Design review of the part built by this model. Coordinates are the model's own, in mm. Round coordinates to 2 decimals unless told otherwise and drop trailing zeros. Order: outer loops, then holes, each group sorted by start corner. A loop starts at its lowest first (then second) coordinate and runs counter-clockwise, first axis right, second up. Notation, with made-up numbers: (-7.5, -10.75) - (29.5, -10.75) arc R21 ccw to (29.5, 2.25) - close; hole circle Ø3 at (53.5, -29). An arc over 180 degrees is marked (long way). Write item = value, one per line.
from build123d import *

# Parameters (mm, degrees)
F0_W    = 4
F0_H    = 2.5
F2_SIZE = 0.4


with BuildPart() as f1:
    # F0 (on Front) → F1 (revolve)
    with BuildSketch(Plane.XZ):
        with Locations((2, 3.75)):
            Rectangle(F0_W, F0_H)
    revolve(axis=Axis((1.361359, 0, 0), (1, 0, 0)))

    # F2
    f2_edges = [f1.edges().sort_by_distance(p)[0] for p in [
        (0, 0, -2.5),
        (4, 0, -2.5),
        (2, 0, 2.5),
        (4, 0, -5),
        (0, 0, -5),
        (2, 0, 5),
    ]]
    chamfer(f2_edges, length=F2_SIZE)


solid = f1.part
Item 1: For line 1 along Z through (x, y) = (1.1, 0); line 2 along Y through (x, z) = (2.5, 2.25), list the stretches that pass through material, from the lowest coordinate up. Write a range as [from, to].
Data:
line_1 = [-5, -2.5], [2.5, 5]
line_2 = [-4.47, -1.09], [1.09, 4.47]
Item 2: The part is to be moulded in two halves that separate along Z. For faces 1 (the face through (2.02, 2.44, -0.54)), 2 (the face through (4, 3, -1)), 3 (the face through (2.02, 4.88, -1.08)), say which applies: +Z half, -Z half, draft (parallel to the pull), parting line (faces both ways), or undercut.
Data:
face_1 = undercut
face_2 = draft
face_3 = parting line
Item 3: Take a section at C-C, the plane x = 1.8. State the section outline as (y, z) points, and give its area (3 significant figures).
Data:
outline = circle Ø10 at (0, 0); hole circle Ø5 at (0, 0)
area = 58.9 mm2
Item 4: Take a section at A-A, the plane y = 0. State the section outline as (x, z) points.
Data:
outline = (0, -4.6) - (0.4, -5) - (3.6, -5) - (4, -4.6) - (4, -2.9) - (3.6, -2.5) - (0.4, -2.5) - (0, -2.9) - close; (0, 2.9) - (0.4, 2.5) - (3.6, 2.5) - (4, 2.9) - (4, 4.6) - (3.6, 5) - (0.4, 5) - (0, 4.6) - close
Item 5: Insertion check: P1, Ø6, axis at y = 0, z = 0, coming from the +X side; P2, Ø2, axis at x = 3.5, z = 3, coming from the +Y side. Each pin has a flat end and moves straight along its axis. Give the tip position at first contact, or say it passes through.
Data:
P1 = 4
P2 = 4.58
